```python
from build123d import *

# Parameters (mm, degrees)
SKETCH1_R               = 17.5
BOSS_EXTRUDE1_DEPTH     = 47
CUT_EXTRUDE1_START      = -7
SKETCH2_R               = 17.5
SKETCH2_R_2             = 15
CUT_EXTRUDE1_DEPTH      = 7
CUT_EXTRUDE2_DEPTH      = 54.117793629
CUT_EXTRUDE3_REACH      = 59.684
CUT_EXTRUDE3_END_RADIUS = 17.5
SKETCH4_R               = 3


with BuildPart() as part:
    # Sketch1 → Boss-Extrude1 (new body)
    with BuildSketch(Plane(origin=(0, 0, 0), x_dir=(1, 0, 0), z_dir=(0, 1, 0))):
        with Locations(Location((0, 0, 0), (0, 0, 270))):
            Circle(SKETCH1_R)
    extrude(amount=BOSS_EXTRUDE1_DEPTH)

    # Sketch2 → Cut-Extrude1 (cut)
    with BuildSketch(Plane(origin=(0, 47, 0), x_dir=(1, 0, 0), z_dir=(0, 1, 0)).offset(CUT_EXTRUDE1_START)):
        with Locations(Location((0, 0, 0), (0, 0, 270))):
            Circle(SKETCH2_R)
        with Locations(Location((0, 0, 0), (0, 0, 270))):
            Circle(SKETCH2_R_2, mode=Mode.SUBTRACT)
    extrude(amount=CUT_EXTRUDE1_DEPTH, mode=Mode.SUBTRACT)

    # Sketch3 → Cut-Extrude2 (cut, through all)
    with BuildSketch(Plane.XZ):
        with BuildLine():
            Line((0, 11), (-3, 11))
            Line((-3, 11), (-3, 8.485281374))
            ThreePointArc((-3, 8.485281374), (0, -9), (3, 8.485281374))
            Line((3, 8.485281374), (3, 11))
            Line((3, 11), (0, 11))
        make_face()
    extrude(amount=-CUT_EXTRUDE2_DEPTH, mode=Mode.SUBTRACT)

    # Cut-Extrude3: up to this cylinder (the profile starts inside it)
    cut_extrude3_end = Plane(origin=(0, 15, 0), z_dir=(0, -1, 0)) * Cylinder(CUT_EXTRUDE3_END_RADIUS, 167.368, mode=Mode.PRIVATE)
    # Sketch4 → Cut-Extrude3 (cut, up to the surface)
    with BuildSketch(Plane(origin=(0, 0, 11), x_dir=(-1, 0, 0), z_dir=(0, 0, -1)), mode=Mode.PRIVATE) as cut_extrude3_sk1:
        with Locations((0, 9)):
            Circle(SKETCH4_R)
    cut_extrude3_tool1 = extrude(cut_extrude3_sk1.sketch, amount=-CUT_EXTRUDE3_REACH, mode=Mode.PRIVATE) & cut_extrude3_end
    add(cut_extrude3_tool1.solids().sort_by_distance((0, 9, 11))[0], mode=Mode.SUBTRACT)
    # Sketch4 → Cut-Extrude3 (cut, up to the surface)
    with BuildSketch(Plane(origin=(0, 0, 11), x_dir=(-1, 0, 0), z_dir=(0, 0, -1)), mode=Mode.PRIVATE) as cut_extrude3_sk2:
        with Locations((0, 21)):
            Circle(SKETCH4_R)
    cut_extrude3_tool2 = extrude(cut_extrude3_sk2.sketch, amount=-CUT_EXTRUDE3_REACH, mode=Mode.PRIVATE) & cut_extrude3_end
    add(cut_extrude3_tool2.solids().sort_by_distance((0, 21, 11))[0], mode=Mode.SUBTRACT)


solid = part.part
```
Check sheet for the modelled part. Datum: model origin and axes. Units: mm. A direction names the side the tool comes from. Give positions to 0.01 mm unless a question says otherwise; leave off trailing zeros. Order: outer loops, then holes, each group sorted by start corner. A loop starts at its lowest first (then second) coordinate and runs counter-clockwise, first axis right, second up. Notation, with made-up numbers: M 81,39 L 133,39 A18 ccw 133,49 Z; hole C 29,14 d9. An arc over 180 degrees is marked long. Answer in a Markdown table with one row per item.
1) Cross-section at D-D, the plane x = -7.5. Enter the section's corners in (y, z), plus the area to 3 significant figures.
Filled sheet:
| item | result |
|---|---|
| outline | M 0,-15.81 L 40,-15.81 L 40,-12.99 L 47,-12.99 L 47,-4.97 L 0,-4.97 Z; M 0,4.97 L 47,4.97 L 47,12.99 L 40,12.99 L 40,15.81 L 0,15.81 Z |
| area | 979 mm2 |
2) Access from +Z, -Z, +X, -X, +Y, -Y to the whole of each face (thin tool, end or side, straight path). Record for faces 5 (the flat face through (-8, 0, 8)), 6 (the cylindrical face through (3, 9, 14)), 7 (the flat face through (3, 23, 10)).
Filled sheet:
| item | result |
|---|---|
| face 5 | +Z, -Z, +X, -X, -Y |
| face 6 | +Z |
| face 7 | +Y, -Y |
3) Cross-section at B-B, the plane z = -6.5. Enter the section's corners in (x, y), plus the area to 3 significant figures.
Filled sheet:
| item | result |
|---|---|
| outline | M -16.25,0 L -6.22,0 L -6.22,47 L -13.52,47 L -13.52,40 L -16.25,40 Z; M 6.22,0 L 16.25,0 L 16.25,40 L 13.52,40 L 13.52,47 L 6.22,47 Z |
| area | 904 mm2 |
4) Thickness scan on L1, parallel to Y at x = 0, z = 13.25; L2, parallel to X at y = 44.5, z = 0; L3, parallel to X at y = 9, z = 15.25. Record the ranges inside material, lowest first. Write a range as [from, to].
Filled sheet:
| item | result |
|---|---|
| L1 | y = [0, 6], [12, 18], [24, 47] |
| L2 | x = [-15, -9], [9, 15] |
| L3 | x = [-8.58, -3], [3, 8.58] |
5) Gauge pin test, flat ends, axial feed: P1, Ø3, axis at x = -3.5, y = 15.5, coming from the +Z side; P2, Ø10, axis at x = -2.5, z = -1.5, coming from the -Y side; P3, Ø3, axis at x = -7, y = 23, coming from the +Z side; P4, Ø12, axis at x = 10.5, y = 32, coming from the -Z side. Record the tip position at first contact, or that the pin passes through.
Filled sheet:
| item | result |
|---|---|
| P1 | stops at z = 17.39 |
| P2 | passes through |
| P3 | stops at z = 16.61 |
| P4 | stops at z = -16.91 |
6) Release check for a two-part mould opening along X. For faces 1 (the flat face through (0, 3, 11)), 2 (the flat face through (8, 40, 13)), 3 (the cylindrical face through (0.66, 43.451, -14.985)), 4 (the flat face through (0, 15, 11)) record: +X half, -X half, draft (parallel to the pull), parting line (faces both ways), or undercut.
Filled sheet:
| item | result |
|---|---|
| face 1 | undercut |
| face 2 | draft |
| face 3 | parting line |
| face 4 | undercut |
7) Cross-section at A-A, the plane y = 26.5. Enter the section's corners in (x, z).
Filled sheet:
| item | result |
|---|---|
| outline | C 0,0 d35; hole M -3,8.49 A9 ccw long 3,8.49 L 3,11 L -3,11 Z |
8) Cross-section at C-C, the plane x = 0. Enter the section's corners in (y, z).
Filled sheet:
| item | result |
|---|---|
| outline | M 0,-17.5 L 40,-17.5 L 40,-15 L 47,-15 L 47,-9 L 0,-9 Z; M 0,11 L 6,11 L 6,17.5 L 0,17.5 Z; M 12,11 L 18,11 L 18,17.5 L 12,17.5 Z; M 24,11 L 47,11 L 47,15 L 40,15 L 40,17.5 L 24,17.5 Z |
